Verification items for the finished model (mm, model axes). A direction names the side the tool comes from. Give positions to 0.01 mm unless a question says otherwise; leave off trailing zeros. Order: outer loops, then holes, each group sorted by start corner. A loop starts at its lowest first (then second) coordinate and runs counter-clockwise, first axis right, second up. Notation, with made-up numbers: M -5,64 L 3,64 A21 cw 3,77 Z; hole C 38,34.5 d2. An arc over 180 degrees is marked long. Answer as a JSON object with one key per item and string values.
```python
from build123d import *

# Parameters (mm, degrees)
BOSS_EXTRUDE1_DEPTH = 10
BOSS_EXTRUDE2_START = -0.550056
SKETCH2_W           = 10
SKETCH2_H           = 5
BOSS_EXTRUDE2_DEPTH = 10.550056
SKETCH3_R           = 2.1
CUT_EXTRUDE1_DEPTH  = 10
FILLET1_R           = 2


with BuildPart() as part:
    # Sketch1 → Boss-Extrude1 (new body)
    with BuildSketch(Plane.XY):
        with BuildLine():
            Line((-23, 0), (-18, 0))
            ThreePointArc((-18, 0), (0, 18), (18, 0))
            Line((18, 0), (23, 0))
            ThreePointArc((23, 0), (0, 23), (-23, 0))
        make_face()
    extrude(amount=BOSS_EXTRUDE1_DEPTH)

    # Sketch2 → Boss-Extrude2 (add)
    with BuildSketch(Plane.ZY.offset(23).offset(BOSS_EXTRUDE2_START)):
        with Locations((5, 2.5)):
            Rectangle(SKETCH2_W, SKETCH2_H)
    boss_extrude2 = extrude(amount=BOSS_EXTRUDE2_DEPTH)

    # Sketch3 → Cut-Extrude1 (cut)
    with BuildSketch(Plane(origin=(0, 5, 0), x_dir=(1, 0, 0), z_dir=(0, 1, 0))):
        with Locations((-27.72497216, -5)):
            Circle(SKETCH3_R)
    cut_extrude1 = extrude(amount=-CUT_EXTRUDE1_DEPTH, mode=Mode.SUBTRACT)

    # Mirror1: Boss-Extrude2, Cut-Extrude1 across plane
    add(boss_extrude2.mirror(Plane(origin=(0, 0, 0), x_dir=(0, 0, 1), z_dir=(1, 0, 0))))
    add(cut_extrude1.mirror(Plane(origin=(0, 0, 0), x_dir=(0, 0, 1), z_dir=(1, 0, 0))), mode=Mode.SUBTRACT)

    # Fillet1
    fillet1_edges = [part.edges().sort_by_distance(p)[0] for p in [
        (0, 18, 10),
        (-22.449944, 5, 5),
        (-27.724972, 5, 0),
        (-27.724972, 5, 10),
        (-33, 5, 5),
        (-33, 0, 5),
        (25.5, 0, 10),
        (0, 23, 0),
        (0, 23, 10),
        (27.724972, 5, 0),
        (27.724972, 5, 10),
        (33, 5, 5),
        (22.449944, 5, 5),
        (33, 0, 5),
        (25.5, 0, 0),
        (0, 18, 0),
        (-25.5, 0, 0),
        (18, 0, 5),
        (-18, 0, 5),
        (-25.5, 0, 10),
    ]]
    fillet(fillet1_edges, radius=FILLET1_R)


solid = part.part
```
Q1. Material ranges on L1, parallel to X at y = 1.7, z = 5; L2, parallel to X at y = 3.75, z = 5; L3, parallel to Y at x = 29.5, z = 7, recorded low to high.
Resolved:
{"L1": "x = -32.98 to -29.82, -25.62 to -17.92, 17.92 to 25.62, 29.82 to 32.98", "L2": "x = -32.85 to -29.82, -25.62 to -17.61, 17.61 to 25.62, 29.82 to 32.85", "L3": "y = 0 to 5"}
Q2. Release check for a two-part mould opening along Z. For faces 6 (the face through (25.785, 2.535, 5.804)), 7 (the face through (-22.8, 5.4, 5)), 8 (the face through (28.56, 4.4, 0.57)) record: +Z half, -Z half, draft (parallel to the pull), parting line (faces both ways), or undercut.
Resolved:
{"face 6": "undercut", "face 7": "draft", "face 8": "-Z half"}
Q3. Section check B-B on x = 29. Record the cut outline in (y, z), then the cut area to 3 significant figures.
Resolved:
{"outline": "M 0,2 A2 ccw 2,0 L 3,0 A2 ccw 5,2 L 5,3.33 L 0,3.33 Z; M 0,6.67 L 5,6.67 L 5,8 A2 ccw 3,10 L 2,10 A2 ccw 0,8 Z", "area": "29.9 mm²"}
Q4. Gauge pin test, flat ends, axial feed: pin 1 Ø4 at (y, z) = (17.5, 4.5) entering from +X; pin 2 Ø5 at (y, z) = (10.5, 8.5) entering from +X; pin 3 Ø1.5 at (x, y) = (19, 16.5) entering from -Z; pin 4 Ø6 at (y, z) = (14, 3.5) entering from +X. Record the tip position at first contact, or that the pin passes through.
Resolved:
{"pin 1": "stops at x = 16.99", "pin 2": "stops at x = 21.55", "pin 3": "passes through", "pin 4": "stops at x = 20.2"}
Q5. Tool access check on faces 1 (the face through (-25.785, 2.535, 5.804)), 2 (the face through (25.9, 5, 3.6)), 3 (the face through (-18.543, 0.531, 5.042)), 4 (the face through (-28.56, 4.4, 0.57)), 5 (the face through (-25.9, 5, 3.6)). Record the directions out of +Z, -Z, +X, -X, +Y, -Y that give a thin tool (end or side, any length) a straight path to the whole face; none if there is none.
Resolved:
{"face 1": "+Y, -Y", "face 2": "+Z, -Z, +X, +Y", "face 3": "+Z, -Z, -Y", "face 4": "-Z, -X, +Y", "face 5": "+Z, -Z, -X, +Y"}
Q6. Section check A-A on z = 5. Record the cut outline in (x, y), then the cut area to 3 significant figures.
Resolved:
{"outline": "M -33,2 A2 ccw -31,0 L -29.82,0 L -29.82,5 L -31,5 A2 ccw -33,3 Z; M -25.62,0 L -19.9,0 A2 ccw -17.91,1.8 A18 cw 17.91,1.8 A2 ccw 19.9,0 L 25.62,0 L 25.62,5 L 24,5 A2 cw 22.08,6.44 A23 ccw -22.08,6.44 A2 cw -24,5 L -25.62,5 Z; M 29.82,0 L 31,0 A2 ccw 33,2 L 33,3 A2 ccw 31,5 L 29.82,5 Z", "area": "378 mm²"}
